Geometry check sheet. Reference: the model listing, model coordinates, mm. Coordinates: 2 decimals unless noted, no trailing zeros. Loops run counter-clockwise (first coordinate to the right, second up) from the corner with the lowest first, then second, coordinate; pieces in that order, holes last.
from build123d import *

# Parameters (mm, degrees)
BOSS_EXTRUDE1_DEPTH = 2


with BuildPart() as part:
    # Sketch1 → Boss-Extrude1 (new body)
    with BuildSketch(Plane(origin=(0, 0, 0), x_dir=(1, 0, 0), z_dir=(0, 1, 0))):
        with BuildLine():
            Line((0, 0), (20, 0))
            Line((20, 0), (20, -20))
            Line((20, -20), (648.38, -20))
            Line((648.38, -20), (648.38, 0))
            Line((648.38, 0), (668.38, 0))
            Line((668.38, 0), (668.38, 153.21))
            Line((668.38, 153.21), (648.38, 153.21))
            Line((648.38, 153.21), (648.38, 173.21))
            Line((648.38, 173.21), (494.944943633, 173.21))
            Line((494.944943633, 173.21), (494.944943633, 153.21))
            Line((494.944943633, 153.21), (474.944943633, 153.21))
            ThreePointArc((474.944943633, 153.21), (149.385371312, 91.815127637), (296.9, 388.45935867))
            Line((296.9, 388.45935867), (409.658335612, 388.45935867))
            Line((409.658335612, 388.45935867), (409.658335612, 430.45935867))
            Line((409.658335612, 430.45935867), (121.389532072, 430.45935867))
            Line((121.389532072, 430.45935867), (20, 297))
            Line((20, 297), (20, 257))
            Line((20, 257), (0, 257))
            Line((0, 257), (0, 0))
        make_face()
    extrude(amount=BOSS_EXTRUDE1_DEPTH)


solid = part.part
1) Section check A-A on x = 201. Record the cut outline in (y, z), and give its area (3 significant figures).
Data:
outline: (0, -430.46) - (2, -430.46) - (2, -361.66) - (0, -361.66) - close; (0, -45.26) - (2, -45.26) - (2, 20) - (0, 20) - close
area: 268 mm2
2) Material ranges on probe 1 along Z at (x, y) = (296.9, 1.05); probe 2 along Z at (x, y) = (528, 1.55); probe 3 along X at (y, z) = (1.6, -125), recorded low to high.
Data:
probe 1: z = -430.46 to -388.46, -18.46 to 20
probe 2: z = -173.21 to 20
probe 3: x = 0 to 129.36, 464.44 to 668.38
3) Depth check by flat-ended pin: pin 1 (0.6 mm diameter, centred on y = 1, z = -168, fed in from +X); pin 2 (1 mm diameter, centred on x = 488, y = 1.5, fed in from -Z); pin 3 (1 mm diameter, centred on y = 0.5, z = -256.5, fed in from +X). Enter the tip coordinate at first touch or a pass-through.
Data:
pin 1: stops at x = 648.38
pin 2: stops at z = -153.21
pin 3: stops at x = 119.82
4) Mould release check, pull along Z, two halves, no side actions. Record for faces 1 (the cylindrical face through (152.92, 0.99, -87.29)), 2 (the flat face through (181, 2, -58)), 3 (the flat face through (71.4, 0.99, -364.66)): +Z half, -Z half, draft (parallel to the pull), parting line (faces both ways), or undercut.
Data:
face 1: undercut
face 2: draft
face 3: -Z half
5) Section check D-D on x = 529.5. Record the cut outline in (y, z).
Data:
outline: (0, -173.21) - (2, -173.21) - (2, 20) - (0, 20) - close
6) Section check C-C on z = -73.5. Record the cut outline in (x, y).
Data:
outline: (0, 0) - (165.24, 0) - (165.24, 2) - (0, 2) - close; (428.56, 0) - (668.38, 0) - (668.38, 2) - (428.56, 2) - close
7) Section check B-B on y = 1.1. Record the cut outline in (x, z).
Data:
outline: (0, -257) - (20, -257) - (20, -297) - (121.39, -430.46) - (409.66, -430.46) - (409.66, -388.46) - (296.9, -388.46) arc R185 cw (long way) to (474.94, -153.21) - (494.94, -153.21) - (494.94, -173.21) - (648.38, -173.21) - (648.38, -153.21) - (668.38, -153.21) - (668.38, 0) - (648.38, 0) - (648.38, 20) - (20, 20) - (20, 0) - (0, 0) - close
